Geometry: final body of the model. Coordinates: model frame, mm. Coordinates: 2 decimals unless noted, no trailing zeros. Loops run counter-clockwise (first coordinate to the right, second up) from the corner with the lowest first, then second, coordinate; pieces in that order, holes last. Notation, with made-up numbers: M -33.75,-20 L 6.25,-20 A20 ccw 6.25,1 Z; hole C 58.25,51.25 d4. An arc over 180 degrees is marked long. Write each question's results on one line, items separated by ' | '. Start each with the question number.
from build123d import *

# Parameters (mm, degrees)
SKETCH1_R          = 2.25
BASE_FLANGE1_DEPTH = 4
CUT_EXTRUDE1_REACH = 82.722
SKETCH5_R          = 2.25
CUT_EXTRUDE2_DEPTH = 81.721744282
SKETCH6_R          = 2.25
CUT_EXTRUDE3_DEPTH = 81.721744282
SKETCH7_W          = 5
SKETCH7_H          = 102.679491924
SKETCH7_W_2        = 42.679491924
SKETCH7_H_2        = 5
TAB1_DEPTH         = 4
SKETCH8_R          = 2.25
CUT_EXTRUDE4_DEPTH = 81.721744282
SKETCH9_R          = 2.25
CUT_EXTRUDE5_DEPTH = 81.721744282


# Sheet-metal steps are written as plain solids
with BuildPart() as part:
    # Sketch1 → Base-Flange1 (new body)
    with BuildSketch(Plane(origin=(0, 0, 0), x_dir=(1, 0, 0), z_dir=(0, 1, 0))):
        with BuildLine():
            Line((-30, 0), (-30, 42.679491924))
            ThreePointArc((-30, 42.679491924), (-31.339745962, 47.679491924), (-35, 51.339745962))
            ThreePointArc((-35, 51.339745962), (-37.071067812, 67.071067812), (-21.339745962, 65))
            ThreePointArc((-21.339745962, 65), (-17.679491924, 61.339745962), (-12.679491924, 60))
            Line((-12.679491924, 60), (0, 60))
            Line((0, 60), (12.679491924, 60))
            ThreePointArc((12.679491924, 60), (17.679491924, 61.339745962), (21.339745962, 65))
            ThreePointArc((21.339745962, 65), (37.071067812, 67.071067812), (35, 51.339745962))
            ThreePointArc((35, 51.339745962), (31.339745962, 47.679491924), (30, 42.679491924))
            Line((30, 42.679491924), (30, 0))
            Line((30, 0), (30, -42.679491924))
            ThreePointArc((30, -42.679491924), (31.339745962, -47.679491924), (35, -51.339745962))
            ThreePointArc((35, -51.339745962), (37.071067812, -67.071067812), (21.339745962, -65))
            ThreePointArc((21.339745962, -65), (17.679491924, -61.339745962), (12.679491924, -60))
            Line((12.679491924, -60), (0, -60))
            Line((0, -60), (-12.679491924, -60))
            ThreePointArc((-12.679491924, -60), (-17.679491924, -61.339745962), (-21.339745962, -65))
            ThreePointArc((-21.339745962, -65), (-37.071067812, -67.071067812), (-35, -51.339745962))
            ThreePointArc((-35, -51.339745962), (-31.339745962, -47.679491924), (-30, -42.679491924))
            Line((-30, -42.679491924), (-30, 0))
        make_face()
        with Locations(Location((-30, 60, 0), (0, 0, 270))):
            Circle(SKETCH1_R, mode=Mode.SUBTRACT)
        with Locations(Location((30, 60, 0), (0, 0, 270))):
            Circle(SKETCH1_R, mode=Mode.SUBTRACT)
        with Locations(Location((30, -60, 0), (0, 0, 270))):
            Circle(SKETCH1_R, mode=Mode.SUBTRACT)
        with Locations(Location((-30, -60, 0), (0, 0, 270))):
            Circle(SKETCH1_R, mode=Mode.SUBTRACT)
    extrude(amount=-BASE_FLANGE1_DEPTH)

    # Sketch4 → Cut-Extrude1 (cut, up to next)
    with BuildSketch(Plane(origin=(0, 0, 0), x_dir=(1, 0, 0), z_dir=(0, 1, 0)), mode=Mode.PRIVATE) as cut_extrude1_sk1:
        Polygon((-20, 22), (20, 22), (22, 20), (22, -20), (20, -22), (-20, -22), (-22, -20), (-22, 20), align=None)
    cut_extrude1_tool1 = extrude(cut_extrude1_sk1.sketch, amount=-CUT_EXTRUDE1_REACH, mode=Mode.PRIVATE) & part.part
    add(cut_extrude1_tool1.solids().sort_by_distance((0, 0, 0))[0], mode=Mode.SUBTRACT)

    # Sketch5 → Cut-Extrude2 (cut, through all)
    with BuildSketch(Plane.XZ.offset(4)):
        with Locations(Location((-24.343145751, 54.343145751, 0), (0, 0, 270))):
            Circle(SKETCH5_R)
        with Locations(Location((24.343145751, 54.343145751, 0), (0, 0, 270))):
            Circle(SKETCH5_R)
        with Locations(Location((24.343145751, -54.343145751, 0), (0, 0, 270))):
            Circle(SKETCH5_R)
        with Locations(Location((-24.343145751, -54.343145751, 0), (0, 0, 270))):
            Circle(SKETCH5_R)
    extrude(amount=-CUT_EXTRUDE2_DEPTH, mode=Mode.SUBTRACT)

    # Sketch6 → Cut-Extrude3 (cut, through all)
    with BuildSketch(Plane.XZ.offset(4)):
        with Locations(Location((-27.5, -15, 0), (0, 0, 270))):
            Circle(SKETCH6_R)
        with Locations(Location((-27.5, 15, 0), (0, 0, 270))):
            Circle(SKETCH6_R)
        with Locations(Location((27.5, 15, 0), (0, 0, 270))):
            Circle(SKETCH6_R)
        with Locations(Location((27.5, -15, 0), (0, 0, 270))):
            Circle(SKETCH6_R)
    extrude(amount=-CUT_EXTRUDE3_DEPTH, mode=Mode.SUBTRACT)

    # Sketch7 → Tab1 (add)
    with BuildSketch(Plane(origin=(0, 0, 0), x_dir=(1, 0, 0), z_dir=(0, 1, 0))):
        with Locations((-32.5, 0)):
            Rectangle(SKETCH7_W, SKETCH7_H)
        with Locations((32.5, 0)):
            Rectangle(SKETCH7_W, SKETCH7_H)
        with Locations((0, -62.5)):
            Rectangle(SKETCH7_W_2, SKETCH7_H_2)
        with Locations((0, 62.5)):
            Rectangle(SKETCH7_W_2, SKETCH7_H_2)
    extrude(amount=-TAB1_DEPTH)

    # Sketch8 → Cut-Extrude4 (cut, through all)
    with BuildSketch(Plane.XZ.offset(4)):
        with Locations(Location((-16, 46, 0), (0, 0, 270))):
            Circle(SKETCH8_R)
        with Locations(Location((-16, 30, 0), (0, 0, 270))):
            Circle(SKETCH8_R)
        with Locations(Location((16, 46, 0), (0, 0, 270))):
            Circle(SKETCH8_R)
        with Locations(Location((16, 30, 0), (0, 0, 270))):
            Circle(SKETCH8_R)
        with Locations(Location((16, -30, 0), (0, 0, 90))):
            Circle(SKETCH8_R)
        with Locations(Location((16, -46, 0), (0, 0, 90))):
            Circle(SKETCH8_R)
        with Locations(Location((-16, -30, 0), (0, 0, 90))):
            Circle(SKETCH8_R)
        with Locations(Location((-16, -46, 0), (0, 0, 90))):
            Circle(SKETCH8_R)
    extrude(amount=-CUT_EXTRUDE4_DEPTH, mode=Mode.SUBTRACT)

    # Sketch9 → Cut-Extrude5 (cut, through all)
    with BuildSketch(Plane(origin=(0, 0, 0), x_dir=(1, 0, 0), z_dir=(0, 1, 0))):
        with Locations(Location((0, 57.5, 0), (0, 0, 270))):
            Circle(SKETCH9_R)
        with Locations(Location((0, -57.5, 0), (0, 0, 270))):
            Circle(SKETCH9_R)
    extrude(amount=-CUT_EXTRUDE5_DEPTH, mode=Mode.SUBTRACT)


solid = part.part
Item 1: Section A-A, the plane z = 46. Return loops of the section in (x, y), plus the area to 3 significant figures.
Item 2: Section C-C, the plane z = 15. Return loops of the section in (x, y).
Item 3: Contact query for flat-ended pins moving along their axis: P1, Ø2, axis at y = -3, z = 12.5, coming from the -X side; P2, Ø2, axis at y = -0.5, z = 21.5, coming from the +X side. Output: stop coordinate, or through.
Item 4: Section B-B, the plane x = -6. Return loops of the section in (y, z), plus the area to 3 significant figures.
Item 5: Pull-direction query (Z, two-part tool) for faces 1 (the cylindrical face through (30.099, -1.972, -62.248)), 2 (the cylindrical face through (37.25, -1.97, 66.89)), 3 (the flat face through (0, -2, 65)), 4 (the flat face through (26, -4, -1)); classes: released by +Z, released by -Z, zero draft, split by the parting line, or undercut.
Item 6: Ray query, L1, parallel to X at y = -2, z = 15; L2, parallel to X at y = -3.2, z = -46; L3, parallel to X at y = -0.9, z = -2.5. Return the intervals inside material, ascending. Write a range as [from, to].
Item 7: Section D-D, the plane y = -2.2. Count the separate pieces of the cut face and the enclosed holes in it, plus the area to 3 significant figures.
Solutions:
1) outline: M -35,-4 L -18.25,-4 L -18.25,0 L -35,0 Z; M -13.75,-4 L 13.75,-4 L 13.75,0 L -13.75,0 Z; M 18.25,-4 L 35,-4 L 35,0 L 18.25,0 Z | area: 244 mm²
2) outline: M -35,-4 L -29.75,-4 L -29.75,0 L -35,0 Z; M -25.25,-4 L -22,-4 L -22,0 L -25.25,0 Z; M 22,-4 L 25.25,-4 L 25.25,0 L 22,0 Z; M 29.75,-4 L 35,-4 L 35,0 L 29.75,0 Z
3) P1: stops at x = -35 | P2: stops at x = 35
4) outline: M -4,-65 L 0,-65 L 0,-22 L -4,-22 Z; M -4,22 L 0,22 L 0,65 L -4,65 Z | area: 344 mm²
5) face 1: undercut | face 2: undercut | face 3: released by +Z | face 4: zero draft
6) L1: x = [-35, -29.75], [-25.25, -22], [22, 25.25], [29.75, 35] | L2: x = [-35, -18.25], [-13.75, 13.75], [18.25, 35] | L3: x = [-35, -22], [22, 35]
7) separate pieces: 1 | enclosed holes: 23 | area: 7,280 mm²
